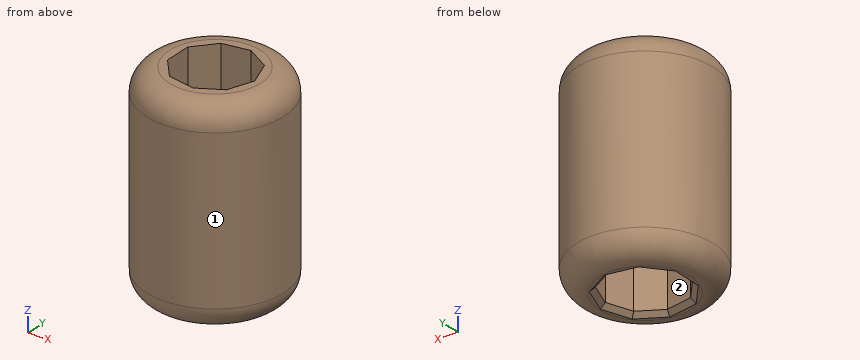
```python
from build123d import *

# Parameters (mm, degrees)
F0_R     = 15
F1_DEPTH = 45
F2_R     = 5
F3_SIZE  = 1


with BuildPart() as f1:
    # F0 (on Top) → F1 (new body)
    with BuildSketch(Plane.XY):
        Circle(F0_R)
        Polygon((-4.488197, 7.405002), (1.321685, 8.557517), (6.513136, 5.705876), (8.657018, 0.184391), (6.750185, -5.423372), (1.684866, -8.493479), (-4.168821, -7.589393), (-8.07187, -3.134146), (-8.198001, 2.787603), align=None, mode=Mode.SUBTRACT)
    extrude(amount=F1_DEPTH)

    # F2
    f2_edges = [f1.edges().sort_by_distance(p)[0] for p in [
        (-15, 0, 45),
        (-15, 0, 0),
    ]]
    fillet(f2_edges, radius=F2_R)

    # F3
    f3_edges = [f1.edges().sort_by_distance(p)[0] for p in [
        (4.217525, -6.958425, 0),
        (-1.241978, -8.041436, 0),
        (-6.120346, -5.361769, 0),
        (-8.134936, -0.173271, 0),
        (-6.343099, 5.096302, 0),
        (-1.583256, 7.98126, 0),
        (3.917411, 7.131697, 0),
        (7.585077, 2.945134, 0),
        (7.703601, -2.61949, 0),
    ]]
    chamfer(f3_edges, length=F3_SIZE)


solid = f1.part
```
Check sheet for the modelled part. Datum: model origin and axes. Units: mm. Face numbers are marked on the shaded views. Give positions to 0.01 mm unless a question says otherwise; leave off trailing zeros. Order: outer loops, then holes, each group sorted by start corner. A loop starts at its lowest first (then second) coordinate and runs counter-clockwise, first axis right, second up. Notation, with made-up numbers: M 40.5,66.5 L 94.5,66.5 A17 ccw 94.5,77.5 Z; hole C 34.25,68.25 d8. An arc over 180 degrees is marked long. Answer in a Markdown table with one row per item. Add a question column.
Q1. Release check for a two-part mould opening along X. For the marked faces 1 and 2 record: released by +X, released by -X, zero draft, split by the parting line, or undercut.
Q2. Gauge pin test, flat ends, axial feed: pin 1 Ø6 at (y, z) = (6.5, 25) entering from +X; pin 2 Ø1 at (y, z) = (11, 17.5) entering from +X; pin 3 Ø3 at (x, z) = (10.5, 40) entering from +Y. Record the tip position at first contact, or that the pin passes through.
Q3. Thickness scan on L1, parallel to Y at x = 0.5, z = 42; L2, parallel to X at y = -2.75, z = 12; L3, parallel to X at y = 2.75, z = 29. Record the ranges inside material, lowest first.
Q4. Sectioned sample at B-B, the plane x = 0. Record the boundary of the cut face in (y, z).
Q5. Sectioned sample at A-A, the plane z = 20. Record the boundary of the cut face in (x, y) (3 decimals).
Verdict:
| question | item | result |
|---|---|---|
| 1 | face 1 | split by the parting line |
| 1 | face 2 | undercut |
| 2 | pin 1 | x = 14.59 |
| 2 | pin 2 | x = 10.71 |
| 2 | pin 3 | y = 12 |
| 3 | L1 | -14.57 to -8.31, 8.39 to 14.57 |
| 3 | L2 | -14.75 to -8.08, 7.66 to 14.75 |
| 3 | L3 | -14.75 to -8.2, 7.66 to 14.75 |
| 4 | outline | M -15,5 A5 ccw -10,0 L -9.25,0 L -8.23,1 L -8.23,45 L -10,45 A5 ccw -15,40 Z; M 8.3,1 L 9.31,0 L 10,0 A5 ccw 15,5 L 15,40 A5 ccw 10,45 L 8.3,45 Z |
| 5 | outline | C 0,0 d30; hole M -8.198,2.788 L -8.072,-3.134 L -4.169,-7.589 L 1.685,-8.493 L 6.75,-5.423 L 8.657,0.184 L 6.513,5.706 L 1.322,8.558 L -4.488,7.405 Z |
